Design review of the part built by this model. Coordinates are the model's own, in mm. A direction names the side the tool comes from. Give positions to 0.01 mm unless a question says otherwise; leave off trailing zeros. Loops run counter-clockwise (first coordinate to the right, second up) from the corner with the lowest first, then second, coordinate; pieces in that order, holes last. Notation, with made-up numbers: M -34,69.25 L -8,69.25 A9 cw -8,79.25 Z; hole C 80,64.25 d6. An arc over 180 degrees is marked long. Use CSV: the item, a comma, the result in double quotes.
from build123d import *

# Parameters (mm, degrees)
SKETCH1_R           = 17.5
BOSS_EXTRUDE1_DEPTH = 12
SKETCH2_R           = 29
BOSS_EXTRUDE2_DEPTH = 5
SKETCH3_R           = 12
CUT_EXTRUDE1_DEPTH  = 5
SKETCH4_R           = 10
CUT_EXTRUDE2_DEPTH  = 1
CUT_EXTRUDE3_REACH  = 44.732
SKETCH5_R           = 3
BOSS_EXTRUDE3_START = 0.9
SKETCH6_R           = 18.8
SKETCH6_R_2         = 17.5
BOSS_EXTRUDE3_DEPTH = 0.9
CUT_EXTRUDE4_REACH  = 46.396
SKETCH7_R           = 8
SKETCH9_R           = 2.7
CUT_EXTRUDE5_DEPTH  = 10


with BuildPart() as part:
    # Sketch1 → Boss-Extrude1 (new body)
    with BuildSketch(Plane(origin=(0, 0, 0), x_dir=(1, 0, 0), z_dir=(0, 1, 0))):
        with Locations(Location((0, 0, 0), (0, 0, 270))):
            Circle(SKETCH1_R)
    extrude(amount=BOSS_EXTRUDE1_DEPTH)

    # Sketch2 → Boss-Extrude2 (add)
    with BuildSketch(Plane(origin=(0, 12, 0), x_dir=(1, 0, 0), z_dir=(0, 1, 0))):
        with Locations(Location((0, 0, 0), (0, 0, 270))):
            Circle(SKETCH2_R)
    extrude(amount=BOSS_EXTRUDE2_DEPTH)

    # Sketch3 → Cut-Extrude1 (cut)
    with BuildSketch(Plane(origin=(0, 17, 0), x_dir=(1, 0, 0), z_dir=(0, 1, 0))):
        with Locations(Location((0, 0, 0), (0, 0, 270))):
            Circle(SKETCH3_R)
    extrude(amount=-CUT_EXTRUDE1_DEPTH, mode=Mode.SUBTRACT)

    # Sketch4 → Cut-Extrude2 (cut)
    with BuildSketch(Plane(origin=(0, 12, 0), x_dir=(1, 0, 0), z_dir=(0, 1, 0))):
        with Locations(Location((0, 0, 0), (0, 0, 270))):
            Circle(SKETCH4_R)
    extrude(amount=-CUT_EXTRUDE2_DEPTH, mode=Mode.SUBTRACT)

    # Sketch5 → Cut-Extrude3 (cut, up to next)
    with BuildSketch(Plane.XZ.offset(-12), mode=Mode.PRIVATE) as cut_extrude3_sk1:
        with Locations(Location((22, 0, 0), (0, 0, 270))):
            Circle(SKETCH5_R)
    cut_extrude3_tool1 = extrude(cut_extrude3_sk1.sketch, amount=-CUT_EXTRUDE3_REACH, mode=Mode.PRIVATE) & part.part
    # Sketch5 → Cut-Extrude3 (cut, up to next)
    with BuildSketch(Plane.XZ.offset(-12), mode=Mode.PRIVATE) as cut_extrude3_sk2:
        with Locations(Location((11, -19.052558883, 0), (0, 0, 270))):
            Circle(SKETCH5_R)
    cut_extrude3_tool2 = extrude(cut_extrude3_sk2.sketch, amount=-CUT_EXTRUDE3_REACH, mode=Mode.PRIVATE) & part.part
    # Sketch5 → Cut-Extrude3 (cut, up to next)
    with BuildSketch(Plane.XZ.offset(-12), mode=Mode.PRIVATE) as cut_extrude3_sk3:
        with Locations(Location((-11, -19.052558883, 0), (0, 0, 270))):
            Circle(SKETCH5_R)
    cut_extrude3_tool3 = extrude(cut_extrude3_sk3.sketch, amount=-CUT_EXTRUDE3_REACH, mode=Mode.PRIVATE) & part.part
    # Sketch5 → Cut-Extrude3 (cut, up to next)
    with BuildSketch(Plane.XZ.offset(-12), mode=Mode.PRIVATE) as cut_extrude3_sk4:
        with Locations(Location((-22, 0, 0), (0, 0, 270))):
            Circle(SKETCH5_R)
    cut_extrude3_tool4 = extrude(cut_extrude3_sk4.sketch, amount=-CUT_EXTRUDE3_REACH, mode=Mode.PRIVATE) & part.part
    # Sketch5 → Cut-Extrude3 (cut, up to next)
    with BuildSketch(Plane.XZ.offset(-12), mode=Mode.PRIVATE) as cut_extrude3_sk5:
        with Locations(Location((-11, 19.052558883, 0), (0, 0, 270))):
            Circle(SKETCH5_R)
    cut_extrude3_tool5 = extrude(cut_extrude3_sk5.sketch, amount=-CUT_EXTRUDE3_REACH, mode=Mode.PRIVATE) & part.part
    # Sketch5 → Cut-Extrude3 (cut, up to next)
    with BuildSketch(Plane.XZ.offset(-12), mode=Mode.PRIVATE) as cut_extrude3_sk6:
        with Locations(Location((11, 19.052558883, 0), (0, 0, 270))):
            Circle(SKETCH5_R)
    cut_extrude3_tool6 = extrude(cut_extrude3_sk6.sketch, amount=-CUT_EXTRUDE3_REACH, mode=Mode.PRIVATE) & part.part
    add(cut_extrude3_tool1.solids().sort_by_distance((22, 12, 0))[0], mode=Mode.SUBTRACT)
    add(cut_extrude3_tool2.solids().sort_by_distance((11, 12, -19.052559))[0], mode=Mode.SUBTRACT)
    add(cut_extrude3_tool3.solids().sort_by_distance((-11, 12, -19.052559))[0], mode=Mode.SUBTRACT)
    add(cut_extrude3_tool4.solids().sort_by_distance((-22, 12, 0))[0], mode=Mode.SUBTRACT)
    add(cut_extrude3_tool5.solids().sort_by_distance((-11, 12, 19.052559))[0], mode=Mode.SUBTRACT)
    add(cut_extrude3_tool6.solids().sort_by_distance((11, 12, 19.052559))[0], mode=Mode.SUBTRACT)

    # Sketch6 → Boss-Extrude3 (add)
    with BuildSketch(Plane.XZ.offset(-12).offset(BOSS_EXTRUDE3_START)):
        with Locations(Location((0, 0, 0), (0, 0, 90))):
            Circle(SKETCH6_R)
        with Locations(Location((0, 0, 0), (0, 0, 270))):
            Circle(SKETCH6_R_2, mode=Mode.SUBTRACT)
    extrude(amount=-BOSS_EXTRUDE3_DEPTH)

    # Sketch7 → Cut-Extrude4 (cut, up to next)
    with BuildSketch(Plane.XZ, mode=Mode.PRIVATE) as cut_extrude4_sk1:
        with Locations(Location((0, 0, 0), (0, 0, 270))):
            Circle(SKETCH7_R)
    cut_extrude4_tool1 = extrude(cut_extrude4_sk1.sketch, amount=-CUT_EXTRUDE4_REACH, mode=Mode.PRIVATE) & part.part
    add(cut_extrude4_tool1.solids().sort_by_distance((0, 0, 0))[0], mode=Mode.SUBTRACT)

    # Sketch9 → Cut-Extrude5 (cut)
    with BuildSketch(Plane.XZ):
        with Locations(Location((0, 12.75, 0), (0, 0, 270))):
            Circle(SKETCH9_R)
        with Locations(Location((11.041823898, 6.375, 0), (0, 0, 270))):
            Circle(SKETCH9_R)
        with Locations(Location((11.041823898, -6.375, 0), (0, 0, 270))):
            Circle(SKETCH9_R)
        with Locations(Location((0, -12.75, 0), (0, 0, 270))):
            Circle(SKETCH9_R)
        with Locations(Location((-11.041823898, -6.375, 0), (0, 0, 270))):
            Circle(SKETCH9_R)
        with Locations(Location((-11.041823898, 6.375, 0), (0, 0, 270))):
            Circle(SKETCH9_R)
    extrude(amount=-CUT_EXTRUDE5_DEPTH, mode=Mode.SUBTRACT)


solid = part.part
(1) Wall thickness on line 1 along Z through (x, y) = (-10, 1.75); line 2 along Z through (x, y) = (-0.5, 11.25); line 3 along Y through (x, z) = (-13.5, -13): over which ranges is each line inside the solid? List them lowest first. Write a range as [from, to].
A:
line 1,"[-14.36, -8.87], [-3.88, 3.88], [8.87, 14.36]"
line 2,"[-18.79, -9.99], [9.99, 18.79]"
line 3,"[11.1, 17]"
(2) Machinability: for faces 4 (the flat face through (8.2, 11, 0)), 5 (the cylindrical face through (-5.65, 11.54, 17.93)), 6 (the cylindrical face through (-24.93, 14.46, 0.65)), which of the approach directions +Z, -Z, +X, -X, +Y, -Y give a long, thin tool a straight path to every point of the face, cutting with its end or side? Answer none if there is none.
A:
face 4,"+Y"
face 5,"-Y"
face 6,"+Y, -Y"
(3) We need section C-C on y = 14. State the section outline as (x, z) points.
A:
outline,"C 0,0 d58; hole C -22,0 d6; hole C -11,-19.05 d6; hole C -11,19.05 d6; hole C 0,0 d24; hole C 11,-19.05 d6; hole C 11,19.05 d6; hole C 22,0 d6"
(4) We need section D-D on x = 22. State the section outline as (y, z) points.
A:
outline,"M 12,-18.89 L 17,-18.89 L 17,-3 L 12,-3 Z; M 12,3 L 17,3 L 17,18.89 L 12,18.89 Z"
(5) Clearance check with flat-ended pins moving along their axes: P1, Ø5, axis at x = 11.04, z = -6.38, coming from the -Y side; P2, Ø16, axis at x = -2, z = 2.5, coming from the +Y side; P3, Ø2, axis at x = -10, y = 14, coming from the -Z side. State where each tip first meets the part, or that it passes through.
A:
P1,"y = 10"
P2,"y = 12"
P3,"z = -27.57"
(6) We need section A-A on z = 0. Count the separate pieces of the cut face and the enclosed holes in it, then the cut area to 3 significant figures.
A:
separate pieces,"4"
enclosed holes,"0"
area,"336 mm²"
(7) The part is to be moulded in two halves that separate along X. For faces 1 (the flat face through (17, 11.1, 5)), 2 (the cylindrical face through (-10.648, 5.472, -13.887)), 3 (the cylindrical face through (0.811, 4.93, 10.175)), say which applies: released by +X, released by -X, zero draft, split by the parting line, or undercut.
A:
face 1,"zero draft"
face 2,"split by the parting line"
face 3,"undercut"
